Geometry check sheet. Reference: drawing and pictorial views, mm from the part's lowest x, y, z. Coordinates: 2 decimals unless noted, no trailing zeros. Write each loop counter-clockwise with the first axis right and the second up, starting at its lowest first coordinate (ties: lowest second). Pieces come first, ordered by that corner, then holes. Notation, with made-up numbers: (9, 56) - (40, 56) arc R12 ccw to (40, 72) - close; hole circle Ø6 at (74, 30.25). An arc over 180 degrees is marked (long way). Answer as a JSON object with one key per item and string values. Group by question number.
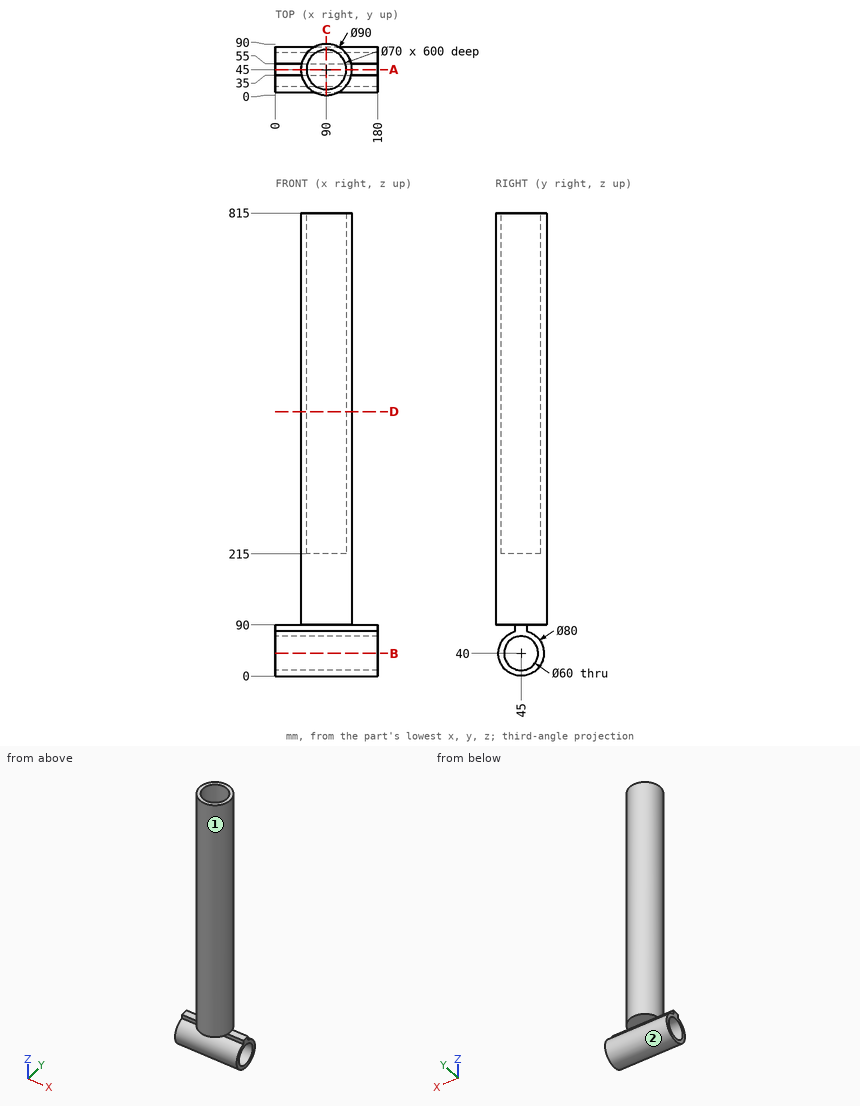
(1) Draft check along Z on the marked faces 1 and 2. Enter one of: +Z half, -Z half, draft (parallel to the pull), parting line (faces both ways), or undercut.
(2) Section check C-C (x = 90). Record the cut outline in (y, z), and give its area (3 significant figures).
(3) Gauge pin test, flat ends, axial feed: pin 1 (8 mm diameter, centred on x = 145.5, y = 80.5, fed in from -Z); pin 2 (6 mm diameter, centred on x = 168, y = 45.5, fed in from +Z); pin 3 (1.5 mm diameter, centred on x = 57.5, y = 30, fed in from -Z). Record the tip position at first contact, or that the pin passes through.
(4) Material ranges on L1, parallel to Z at x = 101, y = 29.5; L2, parallel to Y at x = 57.5, z = 40; L3, parallel to Y at x = 90, z = 445.5, recorded low to high. Write a range as [from, to].
(5) Section check D-D (z = 465.5). Record the cut outline in (x, y).
(6) Section check B-B (z = 40). Record the cut outline in (x, y), and give its area (3 significant figures).
(7) Section check A-A (y = 45). Record the cut outline in (x, z).
Conclusion:
{
 "1": {"face 1": "draft", "face 2": "undercut"},
 "2": {"outline": "(0, 90) - (35, 90) - (35, 78.73) arc R40 ccw (long way) to (55, 78.73) - (55, 90) - (90, 90) - (90, 815) - (80, 815) - (80, 215) - (10, 215) - (10, 815) - (0, 815) - close; hole circle Ø60 at (45, 40)", "area": "25,700 mm^2"},
 "3": {"pin 1": "stops at z = 15.35", "pin 2": "stops at z = 90", "pin 3": "stops at z = 2.62"},
 "4": {"L1": "z = [3.13, 14.31], [65.69, 76.87], [90, 215]", "L2": "y = [5, 15], [75, 85]", "L3": "y = [0, 10], [80, 90]"},
 "5": {"outline": "circle Ø90 at (90, 45); hole circle Ø70 at (90, 45)"},
 "6": {"outline": "(0, 5) - (180, 5) - (180, 15) - (0, 15) - close; (0, 75) - (180, 75) - (180, 85) - (0, 85) - close", "area": "3,600 mm^2"},
 "7": {"outline": "(0, 0) - (180, 0) - (180, 10) - (0, 10) - close; (0, 70) - (180, 70) - (180, 90) - (135, 90) - (135, 815) - (125, 815) - (125, 215) - (55, 215) - (55, 815) - (45, 815) - (45, 90) - (0, 90) - close"}
}
